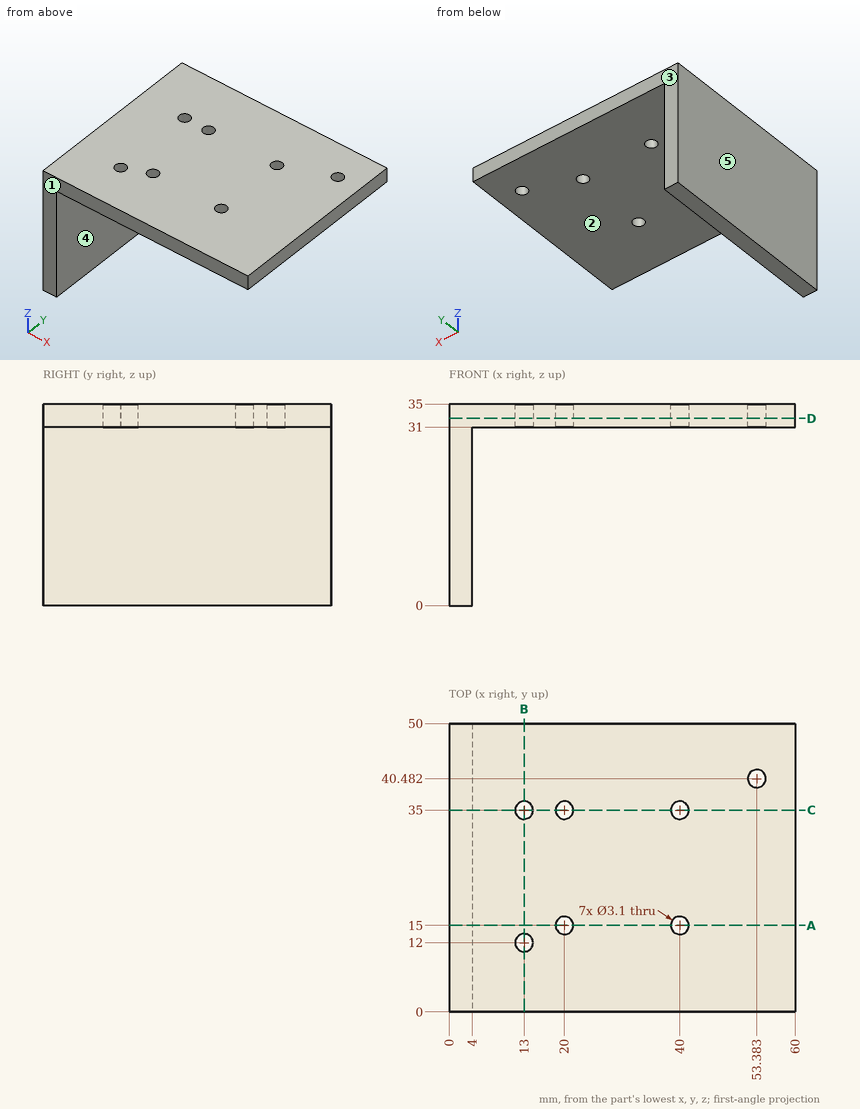
Study the drawing (mm; zero at the part's minimum x, y, z) and answer. A direction names the side the tool comes from. Give positions to 0.01 mm unless a question says otherwise; leave off trailing zeros. Write each loop counter-clockwise with the first axis right and the second up, starting at its lowest first coordinate (ties: lowest second). Pieces come first, ordered by that corner, then holes.
Item 1: Which of the six approach directions +Z, -Z, +X, -X, +Y, -Y give full straight-line access (tool end or side, diameter ignored) to the marked faces 4 and 5?
Item 2: Section B-B, the plane x = 13 is taken. Write down the section's boundary in (y, z).
Item 3: Section D-D, the plane z = 32.5 is taken. Write down the section's boundary in (x, y), plus the area to 3 significant figures.
Item 4: Section A-A, the plane y = 15 is taken. Write down the section's boundary in (x, z), plus the area to 3 significant figures.
Item 5: Determine the mould class of the marked faces 1, 2 and 3 for opening direction Y: released by +Y, released by -Y, zero draft, split by the parting line, or undercut.
Item 6: Section C-C, the plane y = 35 is taken. Write down the section's boundary in (x, z), plus the area to 3 significant figures.
Item 7: Flat-ended cylindrical pins translate along their axes: P1, Ø3, axis at x = 17, z = 28, coming from the -Y side; P2, Ø6, axis at x = 28, y = 9, coming from the -Z side; P3, Ø2, axis at y = 36.5, z = 9.5, coming from the +X side. Find the tip coordinate at first contact, or state that the pin passes through.
Item 8: Find the intervals of material crossed by line 1 along Y through (x, z) = (13, 33.75); line 2 along Y through (x, z) = (20, 31.95); line 3 along Z through (x, y) = (25, 37.5), in increasing order.
Completed:
1. face 4: -Z, +X, +Y, -Y
1. face 5: +Z, -Z, -X, +Y, -Y
2. outline: (0, 31) - (10.45, 31) - (10.45, 35) - (0, 35) - close; (13.55, 31) - (33.45, 31) - (33.45, 35) - (13.55, 35) - close; (36.55, 31) - (50, 31) - (50, 35) - (36.55, 35) - close
3. outline: (0, 0) - (60, 0) - (60, 50) - (0, 50) - close; hole circle Ø3.1 at (13, 12); hole circle Ø3.1 at (13, 35); hole circle Ø3.1 at (20, 15); hole circle Ø3.1 at (20, 35); hole circle Ø3.1 at (40, 15); hole circle Ø3.1 at (40, 35); hole circle Ø3.1 at (53.38, 40.48)
3. area: 2,950 mm2
4. outline: (0, 0) - (4, 0) - (4, 31) - (18.45, 31) - (18.45, 35) - (0, 35) - close; (21.55, 31) - (38.45, 31) - (38.45, 35) - (21.55, 35) - close; (41.55, 31) - (60, 31) - (60, 35) - (41.55, 35) - close
4. area: 339 mm2
5. face 1: released by -Y
5. face 2: zero draft
5. face 3: released by +Y
6. outline: (0, 0) - (4, 0) - (4, 31) - (11.45, 31) - (11.45, 35) - (0, 35) - close; (14.55, 31) - (18.45, 31) - (18.45, 35) - (14.55, 35) - close; (21.55, 31) - (38.45, 31) - (38.45, 35) - (21.55, 35) - close; (41.55, 31) - (60, 31) - (60, 35) - (41.55, 35) - close
6. area: 327 mm2
7. P1: passes through
7. P2: stops at z = 31
7. P3: stops at x = 4
8. line 1: y = 0 to 10.45, 13.55 to 33.45, 36.55 to 50
8. line 2: y = 0 to 13.45, 16.55 to 33.45, 36.55 to 50
8. line 3: z = 31 to 35
